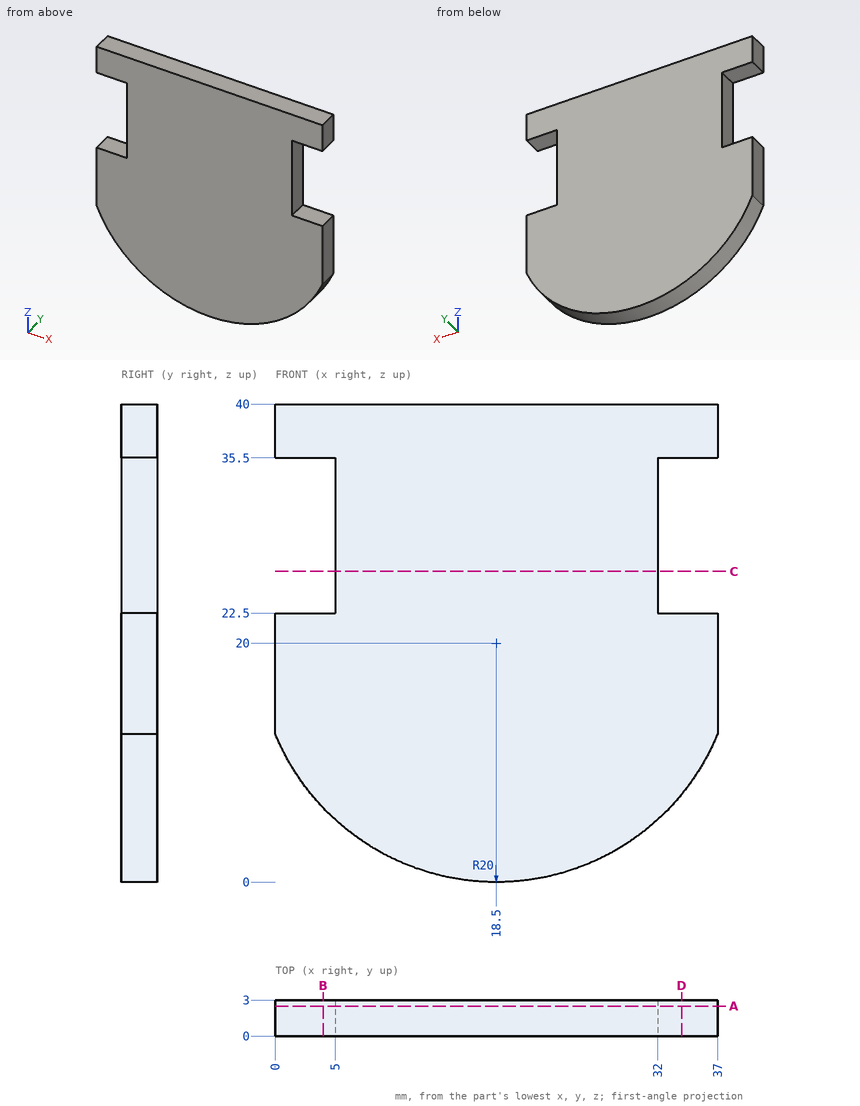
Geometry check sheet. Reference: drawing and pictorial views, mm from the part's lowest x, y, z. Give positions to 0.01 mm unless a question says otherwise; leave off trailing zeros. Write each loop counter-clockwise with the first axis right and the second up, starting at its lowest first coordinate (ties: lowest second). Pieces come first, ordered by that corner, then holes. Notation, with made-up numbers: (77, -5) - (108, -5) arc R25 cw to (108, 13) - close; hole circle Ø10 at (-33, 44). An arc over 180 degrees is marked (long way). Put each result on its own line as item: value.
Q1. Depth check by flat-ended pin: P1, Ø0.9, axis at x = 34.5, y = 1, coming from the -Z side. Enter the tip coordinate at first touch or a pass-through.
Result:
P1: z = 7.42
Q2. Section check D-D on x = 34. Record the cut outline in (y, z), and give its area (3 significant figures).
Result:
outline: (0, 7.36) - (3, 7.36) - (3, 22.5) - (0, 22.5) - close; (0, 35.5) - (3, 35.5) - (3, 40) - (0, 40) - close
area: 58.9 mm2
Q3. Scan lines: probe 1 along Z at (x, y) = (2, 2.85); probe 2 along X at (y, z) = (1.5, 27.5); probe 3 along Z at (x, y) = (33, 2.4). Record each from-to range of solid material in increasing order. Write a range as from..to.
Result:
probe 1: 8.7..22.5, 35.5..40
probe 2: 5..32
probe 3: 6.23..22.5, 35.5..40
Q4. Section check B-B on x = 4. Record the cut outline in (y, z), and give its area (3 significant figures).
Result:
outline: (0, 6.23) - (3, 6.23) - (3, 22.5) - (0, 22.5) - close; (0, 35.5) - (3, 35.5) - (3, 40) - (0, 40) - close
area: 62.3 mm2
Q5. Section check A-A on y = 2.5. Record the cut outline in (x, z).
Result:
outline: (0, 12.4) arc R20 ccw to (37, 12.4) - (37, 22.5) - (32, 22.5) - (32, 35.5) - (37, 35.5) - (37, 40) - (0, 40) - (0, 35.5) - (5, 35.5) - (5, 22.5) - (0, 22.5) - close
Q6. Section check C-C on z = 26. Record the cut outline in (x, y).
Result:
outline: (5, 0) - (32, 0) - (32, 3) - (5, 3) - close
